Geometry check sheet. Reference: drawing and pictorial views, mm from the part's lowest x, y, z. Round coordinates to 2 decimals unless told otherwise and drop trailing zeros. Order: outer loops, then holes, each group sorted by start corner. A loop starts at its lowest first (then second) coordinate and runs counter-clockwise, first axis right, second up.
(1) Sectioned sample at C-C (z = 3). Record the boundary of the cut face in (x, y) (1 decimal).
(2) Release check for a two-part mould opening along X. For the marked faces 1, 2, 3 and 4 record: +X half, -X half, draft (parallel to the pull), parting line (faces both ways), or undercut.
(3) Go/stop test with flat-tipped pins: pin 1 (1.5 mm diameter, centred on x = 15, z = 6.5, fed in from -Y) (1 decimal); pin 2 (3 mm diameter, centred on y = 11, z = 6, fed in from -X); pin 3 (2 mm diameter, centred on x = 15, z = 2, fed in from +Y); pin 4 (1.5 mm diameter, centred on y = 4.5, z = 6.5, fed in from +X). Record where each tip stops, or that it passes through.
(4) Material ranges on line 1 along Y through (x, z) = (11.5, 8.5) (1 decimal); line 2 along X through (y, z) = (12.5, 10.5) (1 decimal); line 3 along Y through (x, z) = (4.75, 8.25) (1 decimal), recorded low to high.
(5) Sectioned sample at B-B (y = 13.25). Record the boundary of the cut face in (x, z) (1 decimal).
(6) Sectioned sample at A-A (x = 12.25). Record the boundary of the cut face in (y, z) (1 decimal).
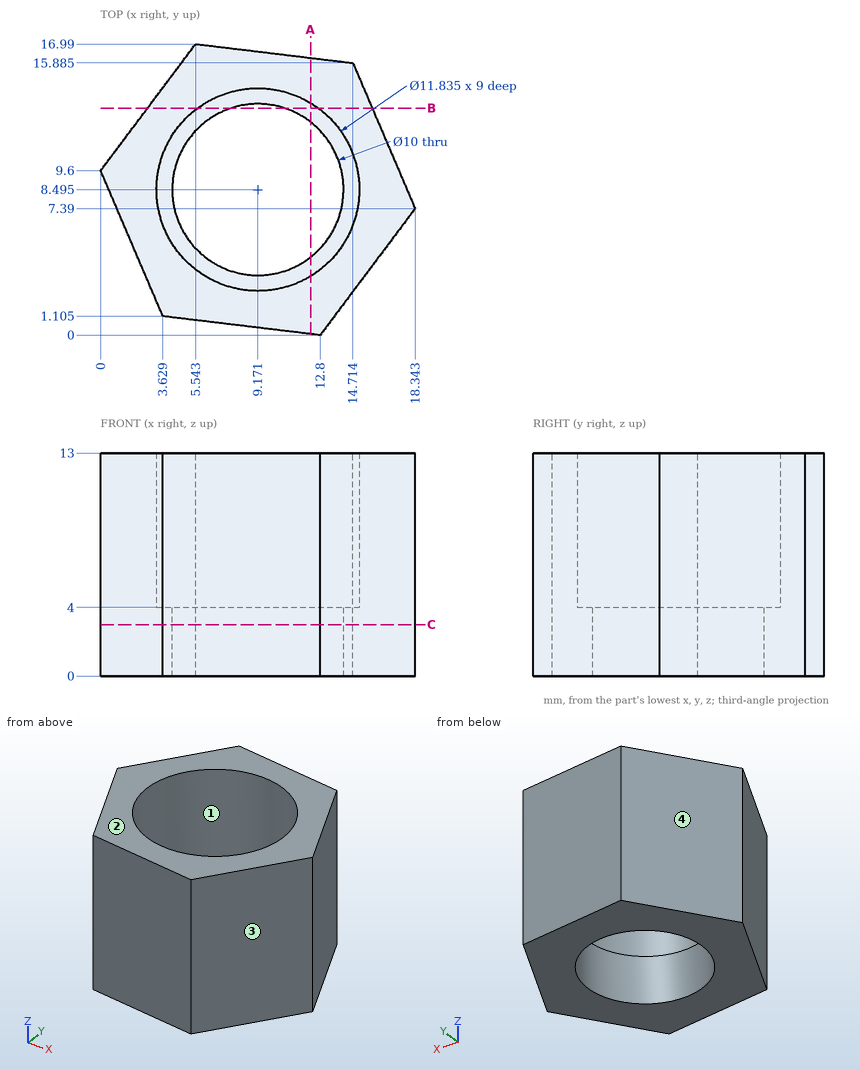
Answer below:
1. outline: (0, 9.6) - (3.6, 1.1) - (12.8, 0) - (18.3, 7.4) - (14.7, 15.9) - (5.5, 17) - close; hole circle Ø10 at (9.2, 8.5)
2. face 1: undercut
2. face 2: draft
2. face 3: +X half
2. face 4: -X half
3. pin 1: stops at y = 1.9
3. pin 2: stops at x = 0
3. pin 3: stops at y = 15.97
3. pin 4: stops at x = 16.74
4. line 1: y = 0.2 to 3.1, 13.9 to 16.3
4. line 2: x = 2.2 to 4.8, 13.5 to 16.2
4. line 3: y = 1 to 4.6, 12.4 to 15.9
5. outline: (2.7, 0) - (7.6, 0) - (7.6, 4) - (5.6, 4) - (5.6, 13) - (2.7, 13) - close; (10.7, 0) - (15.8, 0) - (15.8, 13) - (12.7, 13) - (12.7, 4) - (10.7, 4) - close
6. outline: (0.1, 0) - (4.6, 0) - (4.6, 4) - (3.4, 4) - (3.4, 13) - (0.1, 13) - close; (12.4, 0) - (16.2, 0) - (16.2, 13) - (13.5, 13) - (13.5, 4) - (12.4, 4) - close
